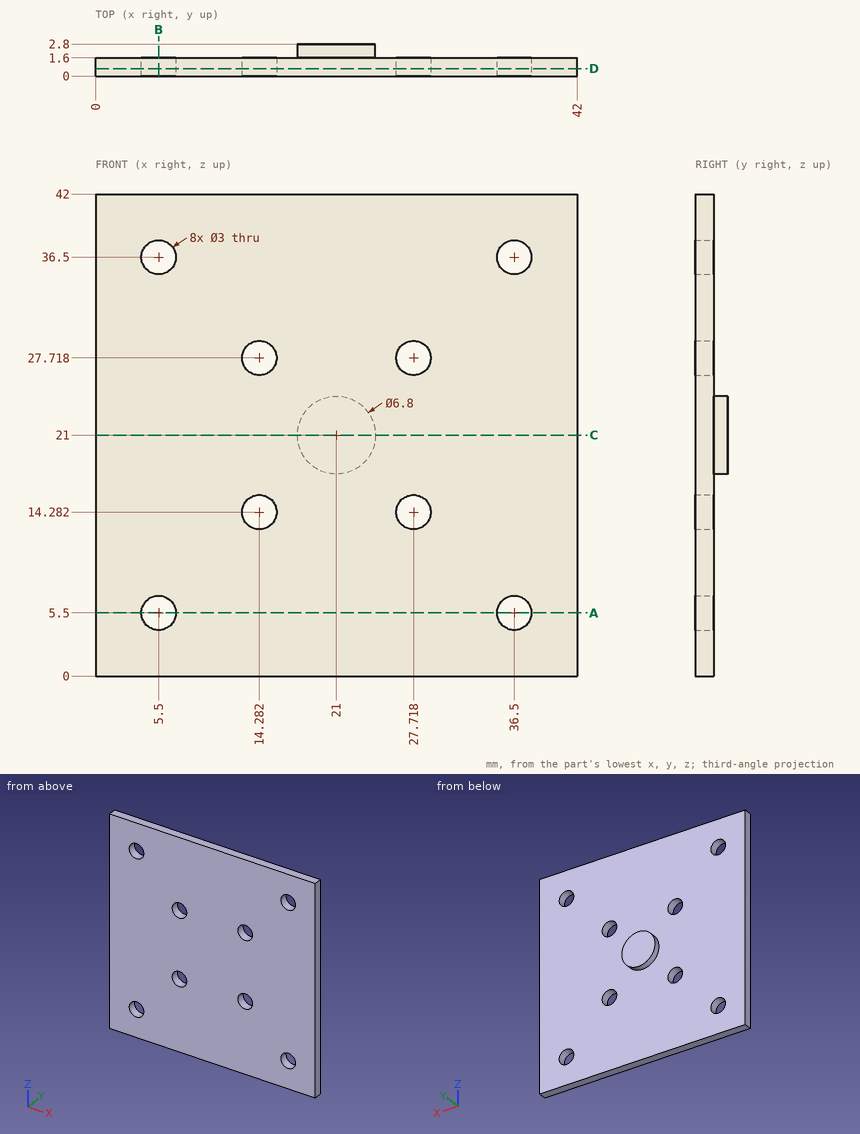
Here's the drawing with two shaded views (mm, measured from the low corner). I have some questions. Round coordinates to 2 decimals unless told otherwise and drop trailing zeros. Loops run counter-clockwise (first coordinate to the right, second up) from the corner with the lowest first, then second, coordinate; pieces in that order, holes last. Notation, with made-up numbers: (27, -10.75) - (66, -10.75) arc R15 cw to (66, 17.25) - close; hole circle Ø5 at (32.5, 1). An arc over 180 degrees is marked (long way). Use CSV: the item, a comma, the result in double quotes. Start each with the question number.
1) If we section it at B-B on x = 5.5: Write out the boundary of the cut face in (y, z).
2) If we section it at A-A on z = 5.5: Write out the boundary of the cut face in (x, y).
3) If we section it at D-D on y = 0.65: Count the separate pieces of the cut face and the enclosed holes in it, plus the area to 3 significant figures.
4) For pin 1 Ø12.5 at (x, z) = (27, 12.5) entering from +Y; pin 2 Ø4 at (x, z) = (27.72, 14.28) entering from -Y, each with a flat end and sliding along its axis, tell me the tip position at first contact or that it passes through.
5) Please list where these lines run through material, in increasing order: probe 1 along X at (y, z) = (0.7, 5.5); probe 2 along Z at (x, y) = (6, 0.4) (1 decimal); probe 3 along Y at (x, z) = (13.5, 16). Write a range as [from, to].
6) If we section it at C-C on z = 21: Write out the boundary of the cut face in (x, y).
Geometry results:
1,outline,"(0, 0) - (1.6, 0) - (1.6, 4) - (0, 4) - close; (0, 7) - (1.6, 7) - (1.6, 35) - (0, 35) - close; (0, 38) - (1.6, 38) - (1.6, 42) - (0, 42) - close"
2,outline,"(0, 0) - (4, 0) - (4, 1.6) - (0, 1.6) - close; (7, 0) - (35, 0) - (35, 1.6) - (7, 1.6) - close; (38, 0) - (42, 0) - (42, 1.6) - (38, 1.6) - close"
3,separate pieces,"1"
3,enclosed holes,"8"
3,area,"1,710 mm2"
4,pin 1,"stops at y = 1.6"
4,pin 2,"stops at y = 0"
5,probe 1,"x = [0, 4], [7, 35], [38, 42]"
5,probe 2,"z = [0, 4.1], [6.9, 35.1], [37.9, 42]"
5,probe 3,"y = [0, 1.6]"
6,outline,"(0, 0) - (42, 0) - (42, 1.6) - (24.4, 1.6) - (24.4, 2.8) - (17.6, 2.8) - (17.6, 1.6) - (0, 1.6) - close"
